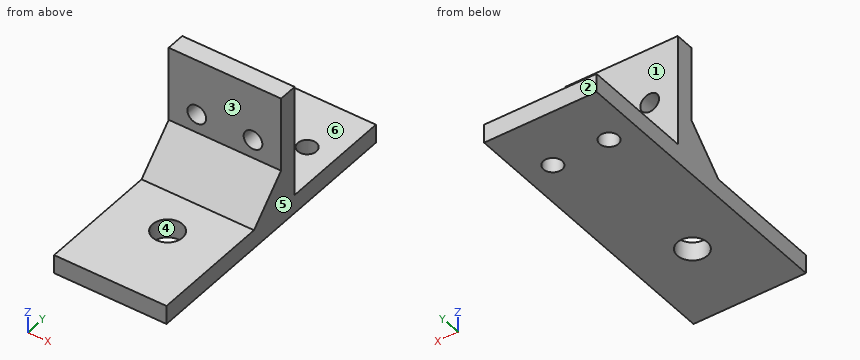
from build123d import *

# Parameters (mm, degrees)
F0_W     = 30
F0_H     = 30
F0_R     = 2.5
F0_H_2   = 5
F0_H_3   = 42.3
F0_R_2   = 4
F1_DEPTH = 5
F2_DEPTH = 35
F4_D     = 5
F4_DEPTH = 12.7
F5_SIZE  = 10


with BuildPart() as f1:
    # F0 (on Top) → F1 (new body)
    with BuildSketch(Plane.XY):
        with Locations((0, 23.65)):
            Rectangle(F0_W, F0_H)
        with Locations((-7.5, 23.65)):
            Circle(F0_R, mode=Mode.SUBTRACT)
        with Locations((7.5, 23.65)):
            Circle(F0_R, mode=Mode.SUBTRACT)
        with Locations((0, 6.15)):
            Rectangle(F0_W, F0_H_2)
        with Locations((0, -17.5)):
            Rectangle(F0_W, F0_H_3)
        with Locations((0, -17.5)):
            Circle(F0_R_2, mode=Mode.SUBTRACT)
    extrude(amount=F1_DEPTH)

    # F0 (on Top) → F2 (join)
    with BuildSketch(Plane.XY):
        with Locations((0, 6.15)):
            Rectangle(F0_W, F0_H_2)
    extrude(amount=F2_DEPTH)

    # F4
    with Locations(Plane.XZ):
        with Locations((-7.5, 20), (7.5, 20)):
            Hole(F4_D / 2, depth=F4_DEPTH)

    # F5
    f5_edges = [f1.edges().sort_by_distance(p)[0] for p in [
        (0, 3.65, 5),
    ]]
    chamfer(f5_edges, length=F5_SIZE)


solid = f1.part
The model under review builds one solid part; all positions refer to its coordinate system, in mm. Face numbers are marked on the shaded views. A direction names the side the tool comes from. Round coordinates to 2 decimals unless told otherwise and drop trailing zeros. Order: outer loops, then holes, each group sorted by start corner. A loop starts at its lowest first (then second) coordinate and runs counter-clockwise, first axis right, second up. Notation, with made-up numbers: (-33, 49.5) -> (-22, 49.5) arc R19 ccw to (-22, 61.5) -> close; hole circle Ø8 at (58, 43). An arc over 180 degrees is marked (long way). Write item = value, one per line. Start each with the question number.
Item 1: For the marked faces 1, 2 and 3, list the 3-axis set-ups (+Z, -Z, +X, -X, +Y, -Y) from which the entire face can be reached by the end or side of a thin tool; tool diameter is ignored.
Item 2: Consider section D-D on y = -17.5. Write out the cut boundary in (x, z), plus the area to 3 significant figures.
Item 3: Mouldability with a two-part tool opening along X and no side actions: class the marked faces 4, 5 and 6 as released by +X, released by -X, zero draft, split by the parting line, or undercut.
Item 4: Consider section B-B on y = 23.65. Write out the cut boundary in (x, z), plus the area to 3 significant figures.
Item 5: For line 1 along Y through (x, z) = (0, 3.2); line 2 along Z through (x, y) = (7.5, 5.1); line 3 along Y through (x, z) = (-7.5, 3.15), list the stretches that pass through material, from the lowest coordinate up.
Item 6: Clearance check with flat-ended pins moving along their axes: pin 1 Ø6.5 at (x, z) = (7.5, 20) entering from -Y; pin 2 Ø15 at (x, z) = (4.5, 16) entering from +Y; pin 3 Ø6.5 at (x, y) = (-7.5, 23.65) entering from +Z; pin 4 Ø2 at (x, z) = (8.5, 19) entering from +Y. State where each tip first meets the part, or that it passes through.
Item 7: Consider section C-C on x = -7.5. Write out the cut boundary in (y, z).
Item 8: Consider section A-A on x = 0. Write out the cut boundary in (y, z).
Conclusion:
q1.face_1 = +Z, +X, -X, +Y
q1.face_2 = +Z, -Z, +X, -X, +Y
q1.face_3 = +Z, +X, -X, -Y
q2.outline = (-15, 0) -> (-4, 0) -> (-4, 5) -> (-15, 5) -> close; (4, 0) -> (15, 0) -> (15, 5) -> (4, 5) -> close
q2.area = 110 mm2
q3.face_4 = undercut
q3.face_5 = released by +X
q3.face_6 = zero draft
q4.outline = (-15, 0) -> (-10, 0) -> (-10, 5) -> (-15, 5) -> close; (-5, 0) -> (5, 0) -> (5, 5) -> (-5, 5) -> close; (10, 0) -> (15, 0) -> (15, 5) -> (10, 5) -> close
q4.area = 100 mm2
q5.line_1 = -38.65 to -21.5, -13.5 to 38.65
q5.line_2 = 0 to 17.5, 22.5 to 35
q5.line_3 = -38.65 to 21.15, 26.15 to 38.65
q6.pin_1 = 3.65
q6.pin_2 = 8.65
q6.pin_3 = 5
q6.pin_4 = through
q7.outline = (-38.65, 0) -> (21.15, 0) -> (21.15, 5) -> (8.65, 5) -> (8.65, 17.5) -> (3.65, 17.5) -> (3.65, 15) -> (-6.35, 5) -> (-38.65, 5) -> close; (3.65, 22.5) -> (8.65, 22.5) -> (8.65, 35) -> (3.65, 35) -> close; (26.15, 0) -> (38.65, 0) -> (38.65, 5) -> (26.15, 5) -> close
q8.outline = (-38.65, 0) -> (-21.5, 0) -> (-21.5, 5) -> (-38.65, 5) -> close; (-13.5, 0) -> (38.65, 0) -> (38.65, 5) -> (8.65, 5) -> (8.65, 35) -> (3.65, 35) -> (3.65, 15) -> (-6.35, 5) -> (-13.5, 5) -> close
